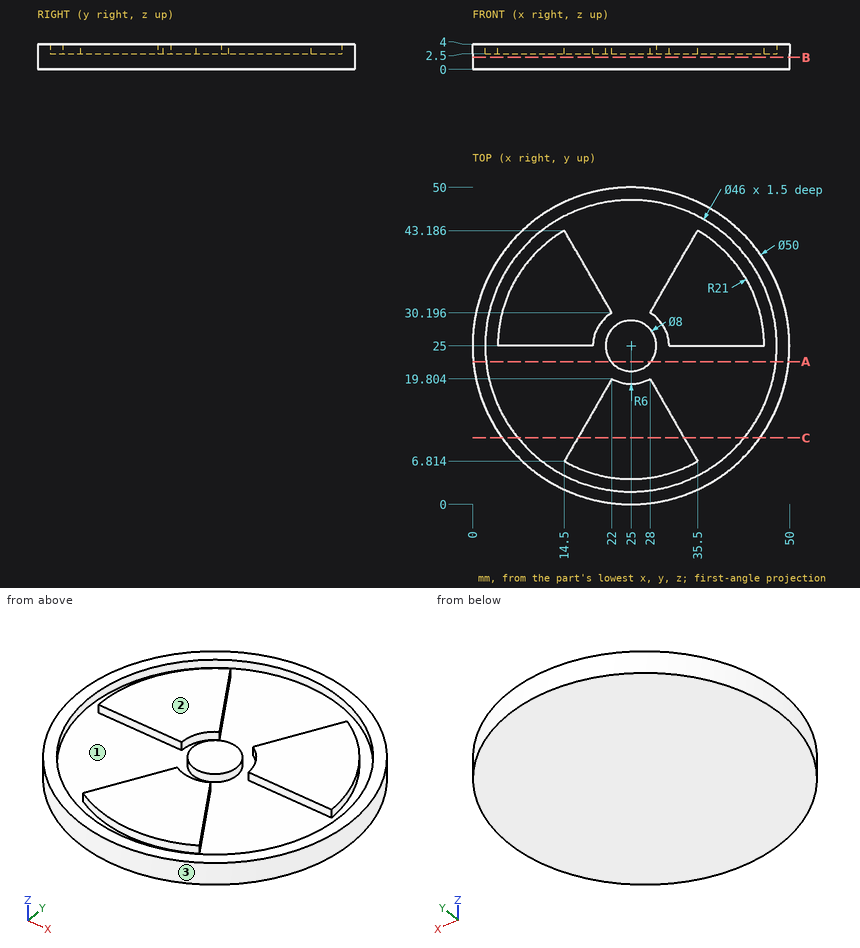
Design review of the part shown in the three views and the two pictorial views. Dimensions are in mm from the part's minimum x, y and z. Round coordinates to 2 decimals unless told otherwise and drop trailing zeros. Order: outer loops, then holes, each group sorted by start corner. A loop starts at its lowest first (then second) coordinate and runs counter-clockwise, first axis right, second up. Notation, with made-up numbers: (2.5, -16.75) -> (43.5, -16.75) arc R25 cw to (43.5, 12.25) -> close; hole circle Ø7 at (29, 5). An arc over 180 degrees is marked (long way). Write item = value, one per line. Start each with the question number.
1) Take a section at B-B on z = 1.9. State the section outline as (x, y) points.
2) Insertion check: pin 1 (2 mm diameter, centred on y = 12.5, z = 2.5, fed in from -X); pin 2 (1 mm diameter, centred on x = 44.5, y = 35, fed in from -Z); pin 3 (0.8 mm diameter, centred on x = 39.5, z = 3.5, fed in from -Y) (1 decimal); pin 4 (1 mm diameter, centred on x = 5.5, z = 1, fed in from -Y). Each pin has a flat end and moves straight along its axis. Give the tip position at first contact, or say it passes through.
3) The part is to be moulded in two halves that separate along Y. For the marked faces 1, 2 and 3, say which applies: +Y half, -Y half, draft (parallel to the pull), parting line (faces both ways), or undercut.
4) Take a section at A-A on y = 22.5. State the section outline as (x, z) points (1 decimal).
5) To check wall thickness, follow line 1 (Y direction, x = 25, z = 3.45); line 2 (Y direction, x = 11.5, z = 3.5) (1 decimal); line 3 (X direction, y = 18, z = 3.55). State the ranges of each line that lie inside material, in increasing order. Write a range as from..to.
6) Take a section at C-C on y = 10.5. State the section outline as (x, z) points (1 decimal).
Verdict:
q1.outline = circle Ø50 at (25, 25)
q2.pin_1 = 2.8
q2.pin_2 = 0
q2.pin_3 = 4.4
q2.pin_4 = 8.75
q3.face_1 = undercut
q3.face_2 = draft
q3.face_3 = parting line
q4.outline = (0.1, 0) -> (49.9, 0) -> (49.9, 4) -> (47.9, 4) -> (47.9, 2.5) -> (28.1, 2.5) -> (28.1, 4) -> (21.9, 4) -> (21.9, 2.5) -> (2.1, 2.5) -> (2.1, 4) -> (0.1, 4) -> close
q5.line_1 = 0..2, 4..19, 21..29, 48..50
q5.line_2 = 4..6.4, 25..41.1, 43.6..46
q5.line_3 = 1..3.09, 20.96..29.04, 46.91..49
q6.outline = (4.6, 0) -> (45.4, 0) -> (45.4, 4) -> (42.9, 4) -> (42.9, 2.5) -> (33.4, 2.5) -> (33.4, 4) -> (16.6, 4) -> (16.6, 2.5) -> (7.1, 2.5) -> (7.1, 4) -> (4.6, 4) -> close
